Could you check a few things on this model? Use its own coordinates, in mm. Face numbers are marked on the shaded views. A direction names the side the tool comes from. Give positions to 0.01 mm unless a question says otherwise; leave off trailing zeros. Order: outer loops, then holes, each group sorted by start corner. A loop starts at its lowest first (then second) coordinate and runs counter-clockwise, first axis right, second up. Notation, with made-up numbers: (-24, -33) - (19, -33) arc R33 cw to (19, 3) - close; hole circle Ø4 at (-12, 10). An arc over 180 degrees is marked (long way). One line per question, with ' | ' between items. Start each with the question number.
1. If we mould it in two halves opening along Y, with no side actions, what happens to the marked faces 4, 5 and 6? For each: released by +Y, released by -Y, zero draft, split by the parting line, or undercut.
2. I need wall thicknesses on probe 1 along X at (y, z) = (30.5, 3); probe 2 along X at (y, z) = (46, 1); probe 3 along X at (y, z) = (35, 9.75). Which ranges of each line are inside material? Lowest first, please. Write a range as from..to.
3. Which directions (+Z, -Z, +X, -X, +Y, -Y) give clear straight access to the entire face, cutting with the end or side of a thin tool? Please do the marked faces 1, 2 and 3.
4. Imagine slicing it at C-C (y = 18.5). Please give me the cut outline in (x, z).
5. For P1, Ø4, axis at x = -90, z = 10.5, coming from the -Y side; P2, Ø4.5, axis at x = -12, z = 7.5, coming from the -Y side; P3, Ø1, axis at y = 21.5, z = 2.5, coming from the +X side; P4, Ø1.5, axis at x = 37.5, z = 11, coming from the +Y side, each with a flat end and sliding along its axis, tell me the tip position at first contact or that it passes through.
6. Imagine slicing it at D-D (z = 7.25). Give the number of separate pieces and of enclosed holes in the cut face, and give its area (3 significant figures).
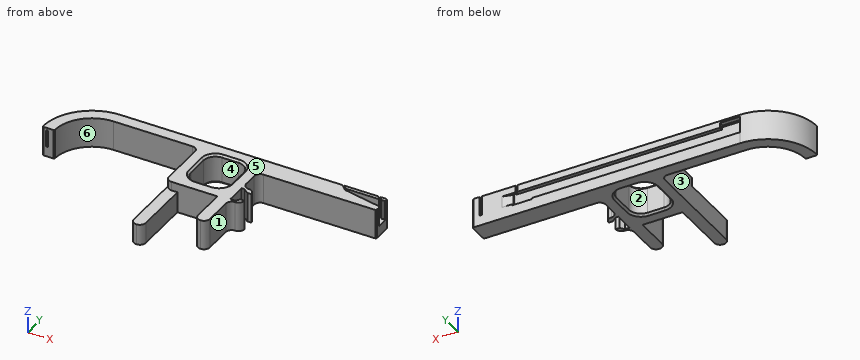
```python
from build123d import *
from OCP.BRepFilletAPI import BRepFilletAPI_MakeChamfer

# Parameters (mm, degrees)
BOSS_EXTRUDE1_DEPTH = 15
BOSS_EXTRUDE2_DEPTH = 15
SKETCH6_W           = 115
SKETCH6_H           = 1
CUT_EXTRUDE2_DEPTH  = 9.85
CUT_EXTRUDE3_DEPTH  = 9.85
CUT_EXTRUDE4_DEPTH  = 9.85
BOSS_EXTRUDE3_DEPTH = 1
CUT_EXTRUDE5_REACH  = 117.913
SKETCH10_W          = 115
SKETCH10_H          = 5.7
SKETCH13_W          = 20.2
SKETCH13_H          = 23
CUT_EXTRUDE6_DEPTH  = 111.121977825
FILLET1_R           = 6
SKETCH14_W          = 6
SKETCH14_H          = 31
CUT_EXTRUDE7_DEPTH  = 4.5
FILLET2_R           = 3
SKETCH16_W          = 10
SKETCH16_H          = 2.5
CUT_EXTRUDE8_DEPTH  = 1.8
CHAMFER1_SIZE       = 0.5
CHAMFER1_SIZE_2     = 0.637377439
CHAMFER2_SIZE       = 1
CHAMFER3_SIZE       = 5
CHAMFER3_SIZE2      = 1.339745962
CUT_EXTRUDE12_REACH = 112.118
CHAMFER4_SIZE       = 0.2
CHAMFER4_SIZE_2     = 0.141421356
SKETCH25_W          = 6
SKETCH25_H          = 12
BOSS_EXTRUDE6_DEPTH = 15
FILLET4_START       = -1
FILLET4_DEPTH       = 16
FILLET4_2_DEPTH     = 15
CUT_EXTRUDE15_DEPTH = 15
CUT_EXTRUDE16_DEPTH = 9.85
CHAMFER5_SIZE       = 0.5
CHAMFER5_SIZE2      = 0.353553391
CHAMFER6_SIZE       = 0.5
SKETCH29_W          = 10
SKETCH29_H          = 0.6
CUT_EXTRUDE17_DEPTH = 2.8


with BuildPart() as part:
    # Sketch3 → Boss-Extrude1 (new body)
    with BuildSketch(Plane.XY):
        Polygon((0, 0), (0, 20.2), (-20.2, 20.2), (-20.2, -10.8), (-26.2, -10.8), (-26.2, 49.2), (-69.1, 49.2), (-69.1, 55.2), (5.9, 55.2), (65.9, 55.2), (65.9, 45.2), (6, 45.2), (6, 0), align=None)
    extrude(amount=BOSS_EXTRUDE1_DEPTH)

    # Sketch4 → Boss-Extrude2 (add)
    with BuildSketch(Plane.XY.offset(15)):
        with BuildLine():
            Line((-88.1, 30.2), (-94.1, 30.2))
            ThreePointArc((-94.1, 30.2), (-86.77766953, 47.87766953), (-69.1, 55.2))
            Line((-69.1, 55.2), (-69.1, 49.2))
            ThreePointArc((-69.1, 49.2), (-82.535028843, 43.635028843), (-88.1, 30.2))
        make_face()
    extrude(amount=-BOSS_EXTRUDE2_DEPTH)

    # Sketch6 → Cut-Extrude2 (cut)
    with BuildSketch(Plane.XY.offset(15)):
        with Locations((-11.6, 52.9)):
            Rectangle(SKETCH6_W, SKETCH6_H)
    extrude(amount=-CUT_EXTRUDE2_DEPTH, mode=Mode.SUBTRACT)

    # Sketch7 → Cut-Extrude3 (cut)
    with BuildSketch(Plane.XY.offset(15)):
        with BuildLine():
            Line((-92.3, 30.2), (-91.3, 30.2))
            ThreePointArc((-91.3, 30.2), (-84.797770542, 45.897770542), (-69.1, 52.4))
            Line((-69.1, 52.4), (-69.1, 53.4))
            ThreePointArc((-69.1, 53.4), (-85.504877324, 46.604877324), (-92.3, 30.2))
        make_face()
    extrude(amount=-CUT_EXTRUDE3_DEPTH, mode=Mode.SUBTRACT)

    # Sketch8 → Cut-Extrude4 (cut)
    with BuildSketch(Plane.XY.offset(15)):
        Polygon((45.9, 53.4), (65.9, 53.4), (65.9, 48.4), (45.9, 52.4), align=None)
    extrude(amount=-CUT_EXTRUDE4_DEPTH, mode=Mode.SUBTRACT)

    # Sketch9 → Boss-Extrude3 (add)
    with BuildSketch(Plane.XY.offset(15)):
        with BuildLine():
            Line((-69.1, 52.4), (45.9, 52.4))
            Line((45.9, 52.4), (45.9, 53.4))
            Line((45.9, 53.4), (-69.1, 53.4))
            ThreePointArc((-69.1, 53.4), (-85.504877324, 46.604877324), (-92.3, 30.2))
            Line((-92.3, 30.2), (-91.3, 30.2))
            ThreePointArc((-91.3, 30.2), (-84.797770542, 45.897770542), (-69.1, 52.4))
        make_face()
    extrude(amount=-BOSS_EXTRUDE3_DEPTH)

    # Cut-Extrude5: up to this face of the body (flat: up to its plane)
    cut_extrude5_end = Plane(part.part.faces().sort_by_distance((-11.6, 52.4, 9.575))[0])
    # Sketch10 → Cut-Extrude5 (cut, up to the picked face)
    with BuildSketch(Plane(origin=(0, 55.2, 0), x_dir=(-1, 0, 0), z_dir=(0, 1, 0)), mode=Mode.PRIVATE) as cut_extrude5_sk1:
        with Locations((11.6, 8.65)):
            Rectangle(SKETCH10_W, SKETCH10_H)
    cut_extrude5_tool1 = split(extrude(cut_extrude5_sk1.sketch, amount=-CUT_EXTRUDE5_REACH, mode=Mode.PRIVATE), bisect_by=cut_extrude5_end, keep=Keep.BOTH, mode=Mode.PRIVATE)
    add(cut_extrude5_tool1.solids().sort_by(Axis((-11.6, 55.2, 8.65), (0, -1, 0)))[0], mode=Mode.SUBTRACT)

    # Sketch13 → Cut-Extrude6 (cut, through all)
    with BuildSketch(Plane.XY.offset(15)):
        with Locations((-10.1, 37.7)):
            Rectangle(SKETCH13_W, SKETCH13_H)
    extrude(amount=-CUT_EXTRUDE6_DEPTH, mode=Mode.SUBTRACT)

    # Fillet1
    fillet1_edges = [part.edges().sort_by_distance(p)[0] for p in [
        (-20.2, 26.2, 7.5),
        (-20.2, 49.2, 7.5),
        (0, 49.2, 7.5),
        (0, 26.2, 7.5),
    ]]
    fillet(fillet1_edges, radius=FILLET1_R)

    # Sketch14 → Cut-Extrude7 (cut)
    with BuildSketch(Plane.XY.offset(15)):
        with Locations((-23.2, 4.7)):
            Rectangle(SKETCH14_W, SKETCH14_H)
    extrude(amount=-CUT_EXTRUDE7_DEPTH, mode=Mode.SUBTRACT)

    # Fillet2
    fillet2_edges = [part.edges().sort_by_distance(p)[0] for p in [
        (-26.2, 49.2, 7.5),
        (6, 45.2, 7.5),
        (-26.2, 20.2, 12.75),
        (6, 0, 7.5),
        (0, 0, 7.5),
        (-20.2, -10.8, 5.25),
        (-26.2, -10.8, 5.25),
    ]]
    fillet(fillet2_edges, radius=FILLET2_R - 0.0001)  # a hair under: the kernel refuses the full size

    # Sketch16 → Cut-Extrude8 (cut)
    with BuildSketch(Plane(origin=(0, 55.2, 0), x_dir=(-1, 0, 0), z_dir=(0, 1, 0))):
        with Locations((64.1, 12.75)):
            Rectangle(SKETCH16_W, SKETCH16_H)
    extrude(amount=-CUT_EXTRUDE8_DEPTH, mode=Mode.SUBTRACT)

    # Chamfer1
    # the kernel refuses this chamfer: 0.637377439, 0.5 mm, written as the material it takes off along each edge
    with BuildSketch(Plane(origin=(65.9, 55.2, -1.285841494), x_dir=(-1, 0, 0), z_dir=(0, 0, 1)), Plane(origin=(65.9, 45.2, -1.285841494), x_dir=(0, 1, 0), z_dir=(0, 0, 1))) as chamfer1_piece_1:
        Polygon((CHAMFER1_SIZE, 0), (0, CHAMFER1_SIZE), (0, 0), align=None)
    extrude(amount=17.571682988, mode=Mode.SUBTRACT)
    with BuildSketch(Plane(origin=(-88.1, 30.2, 16.303301327), x_dir=(-1, 0, 0), z_dir=(0, 0, -1))) as chamfer1_piece_2:
        with BuildLine():
            Line((CHAMFER1_SIZE, 0), (-0.006759226, 0.506759226))
            ThreePointArc((-0.006759226, 0.506759226), (-0.001786833, 0.26056951), (0, 0))
            Line((0, 0), (CHAMFER1_SIZE, 0))
        make_face()
    extrude(amount=17.606602654, mode=Mode.SUBTRACT)
    with BuildSketch(Plane(origin=(-94.1, 30.2, 16.285841494), x_dir=(1, 0, 0), z_dir=(0, 0, -1))) as chamfer1_piece_3:
        with BuildLine():
            Line((CHAMFER1_SIZE, 0), (0.004902903, -0.495097097))
            ThreePointArc((0.004902903, -0.495097097), (0.001296043, -0.254559377), (0, 0))
            Line((0, 0), (CHAMFER1_SIZE, 0))
        make_face()
    extrude(amount=17.571682988, mode=Mode.SUBTRACT)
    with BuildSketch(Plane(origin=(65.9, 53.4, 16.285841494), x_dir=(-1, 0, 0), z_dir=(0, 0, -1))) as chamfer1_piece_4:
        Polygon((CHAMFER1_SIZE, 0), (0, CHAMFER1_SIZE), (0, 0), align=None)
    extrude(amount=11.135841494, mode=Mode.SUBTRACT)
    with BuildSketch(Plane(origin=(65.9, 48.4, 16.646856161), x_dir=(-0.9805806756909208, 0.1961161351381813, 0), z_dir=(0, 0, -1))) as chamfer1_piece_5:
        Polygon((CHAMFER1_SIZE, 0), (-CHAMFER1_SIZE_2 * 0.196116135199, -CHAMFER1_SIZE_2 * 0.980580675997), (0, 0), align=None)
    extrude(amount=11.496856161, mode=Mode.SUBTRACT)

    # Chamfer2
    chamfer2_edges = [part.edges().sort_by_distance(p)[0] for p in [
        (-10.1, 49.2, 15),
        (-10.1, 49.2, 0),
        (0, 37.7, 15),
        (0, 37.7, 0),
        (-10.1, 26.2, 15),
        (-10.1, 26.2, 0),
        (-20.2, 37.7, 15),
        (-20.2, 37.7, 0),
        (-1.757359313, 47.442640687, 15),
        (-1.757359313, 47.442640687, 0),
        (-1.757359313, 27.957359313, 15),
        (-1.757359313, 27.957359313, 0),
        (-18.442640687, 27.957359313, 15),
        (-18.442640687, 27.957359313, 0),
        (-18.442640687, 47.442640687, 15),
        (-18.442640687, 47.442640687, 0),
    ]]
    chamfer(chamfer2_edges, length=CHAMFER2_SIZE)

    # Chamfer3
    chamfer3_edges = [part.edges().sort_by_distance(p)[0] for p in [
        (45.9, 55.2, 8.65),
    ]]
    chamfer3_side = [part.faces().sort_by_distance(p)[0] for p in [
        (64.046661535, 55.2, 7.5),
    ]]
    chamfer(chamfer3_edges, length=CHAMFER3_SIZE, length2=CHAMFER3_SIZE2, reference=chamfer3_side[0])

    # Cut-Extrude12: up to this face of the body (flat: up to its plane)
    cut_extrude12_end = Plane(part.part.faces().sort_by_distance((-5.656799941, 54.307895333, 11.5))[0])
    # Sketch20 → Cut-Extrude12 (cut, up to the picked face)
    with BuildSketch(Plane.XY.offset(15), mode=Mode.PRIVATE) as cut_extrude12_sk1:
        Polygon((45.9, 52.4), (43.1, 55.2), (44.1, 55.2), (45.9, 53.4), align=None)
    cut_extrude12_tool1 = split(extrude(cut_extrude12_sk1.sketch, amount=-CUT_EXTRUDE12_REACH, mode=Mode.PRIVATE), bisect_by=cut_extrude12_end, keep=Keep.BOTH, mode=Mode.PRIVATE)
    add(cut_extrude12_tool1.solids().sort_by(Axis((44.731884, 54.031884, 15), (0, 0, -1)))[0], mode=Mode.SUBTRACT)

    # Chamfer4
    # the kernel refuses this chamfer: 0.2, 0.141421356 mm, written as the material it takes off along each edge
    with BuildSketch(Plane(origin=(44.9, 53.4, 10.985663402), x_dir=(-0.7071067811865297, 0.7071067811865652, 0), z_dir=(0, 0, 1))) as chamfer4_piece_1:
        Polygon((CHAMFER4_SIZE, 0), (CHAMFER4_SIZE_2 * 0.707106782373, CHAMFER4_SIZE_2 * 0.707106782373), (0, 0), align=None)
    extrude(amount=3.014336598, mode=Mode.SUBTRACT)
    with BuildSketch(Plane(origin=(44.1, 55.2, 15.514336598), x_dir=(1, 0, 0), z_dir=(0, 0, -1))) as chamfer4_piece_2:
        Polygon((CHAMFER4_SIZE_2 * 1.00000000168, 0), (CHAMFER4_SIZE * 0.707106781187, CHAMFER4_SIZE * 0.707106781186), (0, 0), align=None)
    extrude(amount=4.528673195, mode=Mode.SUBTRACT)

    # Sketch25 → Boss-Extrude6 (add)
    with BuildSketch(Plane.XY.offset(15)):
        with Locations((9, 26.1)):
            Rectangle(SKETCH25_W, SKETCH25_H)
    extrude(amount=-BOSS_EXTRUDE6_DEPTH)

    # Fillet4: read off the stored shape, not the designer's step
    # Fillet4 outline → Fillet4 (cut)
    with BuildSketch(Plane.XY.offset(FILLET4_START)):
        with BuildLine():
            ThreePointArc((9, 32.1), (11.121320344, 31.221320344), (12, 29.1))
            Line((12, 29.1), (12, 32.1))
            Line((12, 32.1), (9, 32.1))
        make_face()
        with BuildLine():
            ThreePointArc((12, 23.1), (11.121320344, 20.978679656), (9, 20.1))
            Line((9, 20.1), (12, 20.1))
            Line((12, 20.1), (12, 23.1))
        make_face()
    extrude(amount=FILLET4_DEPTH, mode=Mode.SUBTRACT)

    # Fillet4 2 outline → Fillet4 2 (add)
    with BuildSketch(Plane.XY):
        with BuildLine():
            Line((6, 32.1), (9, 32.1))
            ThreePointArc((9, 32.1), (6.878679656, 32.978679656), (6, 35.1))
            Line((6, 35.1), (6, 32.1))
        make_face()
        with BuildLine():
            ThreePointArc((6, 17.1), (6.878679656, 19.221320344), (9, 20.1))
            Line((9, 20.1), (6, 20.1))
            Line((6, 20.1), (6, 17.1))
        make_face()
    extrude(amount=FILLET4_2_DEPTH)

    # Sketch26 → Cut-Extrude15 (cut)
    with BuildSketch(Plane.XY.offset(15)):
        Polygon((12, 29.1), (10, 29.1), (7.402667467, 31.1), (6, 31.1), (6, 21.1), (8.459958458, 21.1), (10, 23.1), (12, 23.1), align=None)
    extrude(amount=-CUT_EXTRUDE15_DEPTH, mode=Mode.SUBTRACT)

    # Sketch27 → Cut-Extrude16 (cut)
    with BuildSketch(Plane.XY.offset(15)):
        Polygon((62.9, 53.4), (61.1, 55.2), (62.1, 55.2), (63.9, 53.4), align=None)
    extrude(amount=-CUT_EXTRUDE16_DEPTH, mode=Mode.SUBTRACT)

    # Chamfer5: one chamfer whose edges measure the first distance from different faces: ONE call of the kernel's chamfer builder (chamfer() names one face for all edges)
    chamfer5_edges_1 = [part.edges().sort_by_distance(p)[0] for p in [
        (62.9, 53.4, 10.075),
    ]]
    chamfer5_side_1 = [part.faces().sort_by_distance(p)[0] for p in [
        (62, 54.3, 10.075),
    ]]
    chamfer5_edges_2 = [part.edges().sort_by_distance(p)[0] for p in [
        (62.1, 55.2, 10.075),
    ]]
    chamfer5_side_2 = [part.faces().sort_by_distance(p)[0] for p in [
        (63, 54.3, 10.075),
    ]]
    chamfer5 = BRepFilletAPI_MakeChamfer(part.part.solid().wrapped)
    for e in chamfer5_edges_1:
        chamfer5.Add(CHAMFER5_SIZE, CHAMFER5_SIZE2, e.wrapped, chamfer5_side_1[0].wrapped)  # the first distance lies on this face
    for e in chamfer5_edges_2:
        chamfer5.Add(CHAMFER5_SIZE, CHAMFER5_SIZE2, e.wrapped, chamfer5_side_2[0].wrapped)  # the first distance lies on this face
    add(Compound.cast(chamfer5.Shape()), mode=Mode.REPLACE)

    # Chamfer6
    chamfer6_edges = [part.edges().sort_by_distance(p)[0] for p in [
        (-7.170710678, 53.4, 14),
        (-11.6, 52.4, 14),
        (-84.797770542, 45.897770542, 14),
        (-85.504877324, 46.604877324, 14),
    ]]
    chamfer(chamfer6_edges, length=CHAMFER6_SIZE - 0.0001)  # a hair under: the kernel refuses the full size

    # Sketch29 → Cut-Extrude17 (cut)
    with BuildSketch(Plane(origin=(0, 55.2, 0), x_dir=(-1, 0, 0), z_dir=(0, 1, 0))):
        with Locations((-40.9, 5.5)):
            Rectangle(SKETCH29_W, SKETCH29_H)
    extrude(amount=-CUT_EXTRUDE17_DEPTH, mode=Mode.SUBTRACT)


solid = part.part
```
Results found:
1) face 4: undercut | face 5: zero draft | face 6: released by -Y
2) probe 1: x = -93.9..-88.3, -26.2..-19.95, -0.25..6, 8.18..11.65 | probe 2: x = -88.47..-79.65, -26.2..-19.51, -0.69..65.9 | probe 3: x = -93.63..-91.8, -90.77..-87.48, -26.2..-20.2, 0..6
3) face 1: +Z, -Z, +X, -Y | face 2: +Z, -Z | face 3: +Z, -Z, -Y
4) outline: (-26.2, 0) - (-20.2, 0) - (-20.2, 10.5) - (-26.2, 10.5) - close; (0, 0) - (6.35, 0) - (6.35, 15) - (0, 15) - close
5) P1: stops at y = 30.2 | P2: stops at y = 20.2 | P3: stops at x = 11.79 | P4: stops at y = 55.2
6) separate pieces: 4 | enclosed holes: 1 | area: 1,660 mm2
